Geometry: see drawing. Coordinates: mm, zero at the bounding-box minimum. Coordinates: 2 decimals unless noted, no trailing zeros. Write each loop counter-clockwise with the first axis right and the second up, starting at its lowest first coordinate (ties: lowest second). Pieces come first, ordered by that corner, then holes. Notation, with made-up numbers: (-9, 7.25) - (43, 7.25) arc R12 cw to (43, 25.25) - close; hole circle Ø2 at (67, 55.25). An arc over 180 degrees is marked (long way). One line per question, with ' | ' between items. Start each with the question number.
1) Section query D-D on x = 23. Return loops of the section in (y, z), and give its area (3 significant figures).
2) Line query: line 1 (X direction, y = 0.2, z = 17) (3 decimals); line 2 (Z direction, x = 27, y = 0.15) (3 decimals); line 3 (Z direction, x = 12, y = 0.3). Output: solid intervals per line, ascending.
3) Section query C-C on z = 10. Return loops of the section in (x, y), and give its area (3 significant figures).
4) Section query B-B on y = 0.15. Return loops of the section in (x, z) (3 decimals), and give its area (3 significant figures).
5) First-contact query: P1, Ø1.5, axis at x = 16.375, z = 16.375, coming from the +Y side. Flat tip, straight axial feed; report the tip coordinate or a pass-through.
6) Section query A-A on x = 26.5. Return loops of the section in (y, z) (3 decimals).
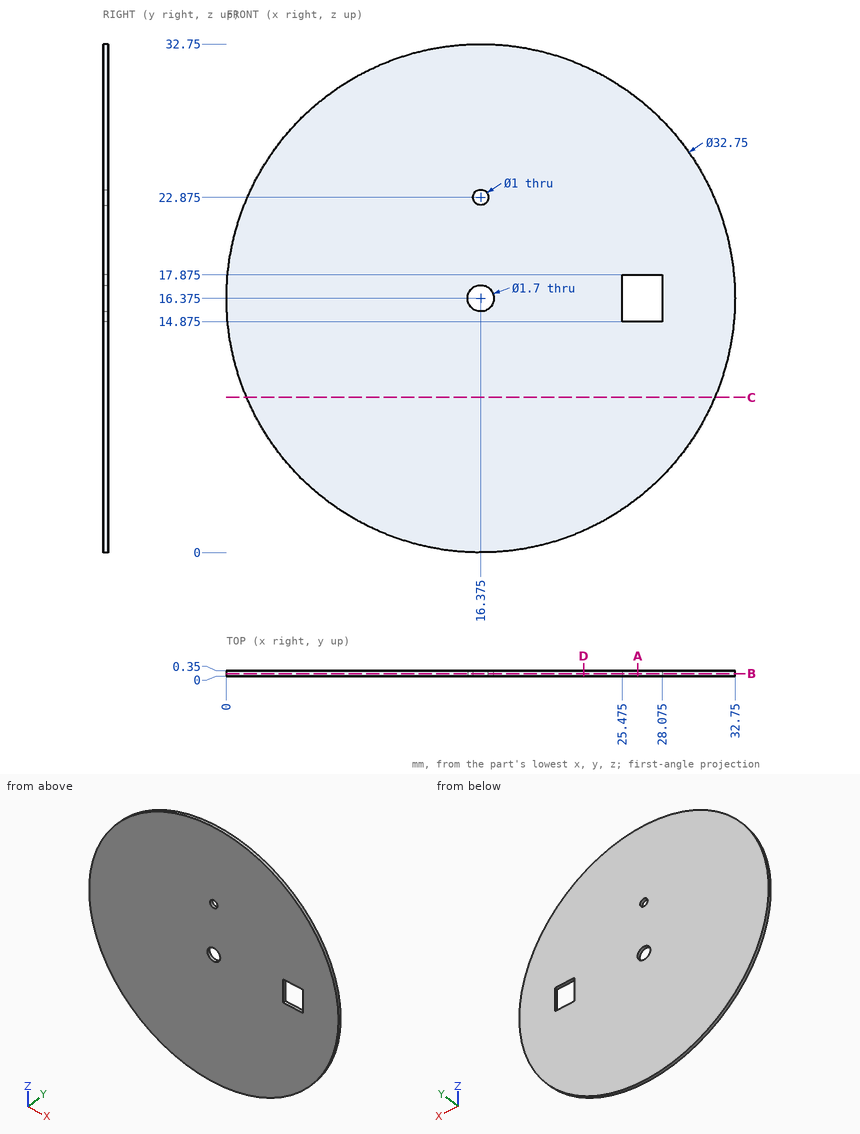
Answer key:
1) outline: (0, 1.4) - (0.35, 1.4) - (0.35, 31.35) - (0, 31.35) - close | area: 10.5 mm²
2) line 1: 0.012 to 15.799, 16.951 to 25.475, 28.075 to 32.738 | line 2: 3.915 to 14.875, 17.875 to 28.835 | line 3: 0.6 to 32.15
3) outline: (1.29, 0) - (31.46, 0) - (31.46, 0.35) - (1.29, 0.35) - close | area: 10.6 mm²
4) outline: circle Ø32.75 at (16.375, 16.375); hole circle Ø1.7 at (16.375, 16.375); hole circle Ø1 at (16.375, 22.875); hole (25.475, 14.875) - (28.075, 14.875) - (28.075, 17.875) - (25.475, 17.875) - close | area: 832 mm²
5) P1: through
6) outline: (0, 3.505) - (0.35, 3.505) - (0.35, 14.875) - (0, 14.875) - close; (0, 17.875) - (0.35, 17.875) - (0.35, 29.245) - (0, 29.245) - close
